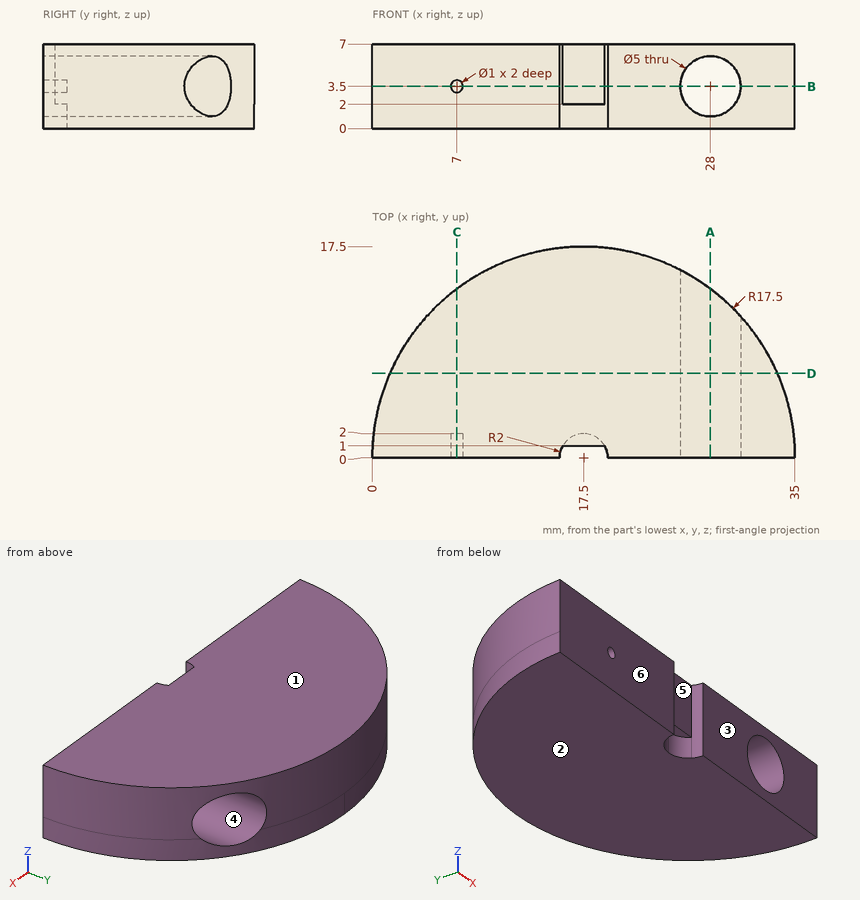
Input: dimensioned drawing with shaded views. Units: mm. Origin: part minimum x, y, z. A direction names the side the tool comes from. Coordinates: 2 decimals unless noted, no trailing zeros. Order: outer loops, then holes, each group sorted by start corner. A loop starts at its lowest first (then second) coordinate and runs counter-clockwise, first axis right, second up.
Item 1: Section query B-B (z = 3.5). Output: boundary loops of the cut face in (x, y), then the cut area to 3 significant figures.
Answer:
outline: (0, 0) - (6.5, 0) - (6.5, 2) - (7.5, 2) - (7.5, 0) - (15.5, 0) arc R2 cw to (15.77, 1) - (19.23, 1) arc R2 cw to (19.5, 0) - (25.5, 0) - (25.5, 15.56) arc R17.5 ccw to start; (30.5, 0) - (35, 0) arc R17.5 ccw to (30.5, 11.72) - close
area: 406 mm2
Item 2: Contact query for flat-ended pins moving along their axis: P1, Ø0.8, axis at x = 17.5, y = 1.5, coming from the -Z side; P2, Ø2, axis at x = 27, z = 5, coming from the +Y side. Output: stop coordinate, or through.
Answer:
P1: stops at z = 2
P2: stops at y = 15.3
Item 3: Material intervals for line 1 along X through (y, z) = (1.3, 3.5); line 2 along X through (y, z) = (1.1, 3.5); line 3 along X through (y, z) = (9.25, 3.5), sorted ascending.
Answer:
line 1: x = 0.05 to 6.5, 7.5 to 25.5, 30.5 to 34.95
line 2: x = 0.03 to 6.5, 7.5 to 25.5, 30.5 to 34.97
line 3: x = 2.64 to 25.5, 30.5 to 32.36
Item 4: Section query D-D (y = 7). Output: boundary loops of the cut face in (x, z), then the cut area to 3 significant figures.
Answer:
outline: (1.46, 0) - (33.54, 0) - (33.54, 7) - (1.46, 7) - close; hole circle Ø5 at (28, 3.5)
area: 205 mm2
Item 5: Draft query along Z for the marked faces 1, 2, 3 and 4. Return one class per face: released by +Z, released by -Z, zero draft, split by the parting line, or undercut.
Answer:
face 1: released by +Z
face 2: released by -Z
face 3: zero draft
face 4: undercut
Item 6: Access query for the marked faces 5 and 6. Directions: +Z, -Z, +X, -X, +Y, -Y. A direction counts if a zero-diameter tool reaches every point of the face in a straight line with its end or side. Return the directions, or none.
Answer:
face 5: +Z, -Z, -Y
face 6: +Z, -Z, +X, -X, -Y
Item 7: Section query A-A (x = 28). Output: boundary loops of the cut face in (y, z).
Answer:
outline: (0, 0) - (14, 0) - (14, 1) - (0, 1) - close; (0, 6) - (14, 6) - (14, 7) - (0, 7) - close
Item 8: Section query C-C (x = 7). Output: boundary loops of the cut face in (y, z), then the cut area to 3 significant figures.
Answer:
outline: (0, 0) - (14, 0) - (14, 7) - (0, 7) - (0, 4) - (2, 4) - (2, 3) - (0, 3) - close
area: 96.0 mm2
